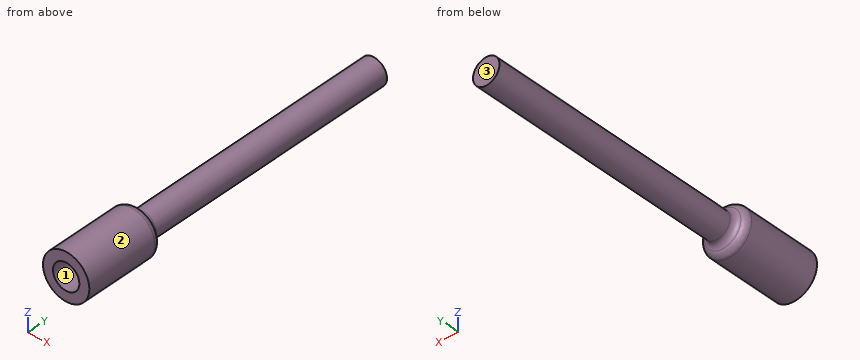
```python
from build123d import *

# Parameters (mm, degrees)
SKETCH_1_R      = 3.5
SKETCH_1_R_2    = 1.99
EXTRUDE_1_DEPTH = 12
SKETCH_2_R      = 2
EXTRUDE_2_DEPTH = 40
FILLET_1_R      = 1
FILLET_2_R      = 1


with BuildPart() as part:
    # Эскиз1 → Вытянуть1 (new body)
    with BuildSketch(Plane(origin=(0, 0, 0), x_dir=(1, 0, 0), z_dir=(0, 1, 0))):
        with Locations(Location((0, 0, 0), (0, 0, 270))):
            Circle(SKETCH_1_R)
        with Locations(Location((0, 0, 0), (0, 0, 270))):
            Circle(SKETCH_1_R_2, mode=Mode.SUBTRACT)
    extrude(amount=EXTRUDE_1_DEPTH)

    # Эскиз2 → Вытянуть2 (add)
    with BuildSketch(Plane(origin=(0, 12, 0), x_dir=(1, 0, 0), z_dir=(0, 1, 0))):
        with Locations(Location((0, 0, 0), (0, 0, 270))):
            Circle(SKETCH_2_R)
    extrude(amount=EXTRUDE_2_DEPTH)

    # Скругление1
    fillet_1_edges = [part.edges().sort_by_distance(p)[0] for p in [
        (0, 12, -2),
    ]]
    fillet(fillet_1_edges, radius=FILLET_1_R)

    # Скругление2
    fillet_2_edges = [part.edges().sort_by_distance(p)[0] for p in [
        (0, 12, -3.5),
    ]]
    fillet(fillet_2_edges, radius=FILLET_2_R)


solid = part.part
```
Here's how the part is built. I have some questions about the finished solid (model axes, mm). Face numbers are marked on the shaded views. Round coordinates to 2 decimals unless told otherwise and drop trailing zeros. Write each loop counter-clockwise with the first axis right and the second up, starting at its lowest first coordinate (ties: lowest second). Pieces come first, ordered by that corner, then holes.
Q1. Will these pins go through, and if not, where does the flat tip stop? P1, Ø1.5, axis at y = 32, z = -0.5, coming from the +X side; P2, Ø1, axis at x = 1, z = 0, coming from the -Y side.
Q2. If we section it at B-B on y = 8: Write out the boundary of the cut face in (x, z), plus the area to 3 significant figures.
Q3. If we section it at A-A on y = 44.5: Write out the boundary of the cut face in (x, z), plus the area to 3 significant figures.
Q4. Please list where these lines run through material, in increasing order: probe 1 along X at (y, z) = (8.5, 0); probe 2 along Y at (x, z) = (1.5, 0.5); probe 3 along Y at (x, z) = (0.75, -2.75).
Q5. If we mould it in two halves opening along Z, with no side actions, what happens to the marked faces 1, 2 and 3? For each: +Z half, -Z half, draft (parallel to the pull), parting line (faces both ways), or undercut.
Answer below:
1. P1: stops at x = 2
1. P2: stops at y = 12
2. outline: circle Ø7 at (0, 0); hole circle Ø3.98 at (0, 0)
2. area: 26.0 mm2
3. outline: circle Ø4 at (0, 0)
3. area: 12.6 mm2
4. probe 1: x = -3.5 to -1.99, 1.99 to 3.5
4. probe 2: y = 12 to 52
4. probe 3: y = 0 to 12
5. face 1: undercut
5. face 2: parting line
5. face 3: draft
